from build123d import *

# Parameters (mm, degrees)
SKETCH1_R           = 1.25
BOSS_EXTRUDE1_DEPTH = 10
CHAMFER1_SIZE       = 0.2


with BuildPart() as part:
    # Sketch1 → Boss-Extrude1 (new body)
    with BuildSketch(Plane(origin=(0, 0, 0), x_dir=(1, 0, 0), z_dir=(0, 1, 0))):
        Polygon((1.443375673, 2.5), (-1.443375673, 2.5), (-2.886751346, 0), (-1.443375673, -2.5), (1.443375673, -2.5), (2.886751346, 0), align=None)
        with Locations(Location((0, 0, 0), (0, 0, 270))):  # turned: the seam where the file's is
            Circle(SKETCH1_R, mode=Mode.SUBTRACT)
    extrude(amount=BOSS_EXTRUDE1_DEPTH)

    # Chamfer1
    chamfer1_edges = [part.edges().sort_by_distance(p)[0] for p in [
        (0, 0, -1.25),
        (0, 10, -1.25),
    ]]
    chamfer(chamfer1_edges, length=CHAMFER1_SIZE)

    # Sketch2 → Cut-Revolve1 (revolve, cut)
    with BuildSketch(Plane.XY, mode=Mode.PRIVATE) as cut_revolve1_sk:
        Polygon((2.386751346, 10), (2.886751346, 9.5), (2.886751346, 10), align=None)
        Polygon((2.386751346, 0), (2.886751346, 0), (2.886751346, 0.5), align=None)
    revolve(cut_revolve1_sk.sketch.rotate(Axis((0, 0, 0), (0, 1, 0)), 270), axis=Axis((0, 0, 0), (0, 1, 0)), mode=Mode.SUBTRACT)  # turned: the seam where the file's is


solid = part.part
Read the model definition and answer for the solid it produces. Units are mm, in the model's axes. Coordinates: 2 decimals unless noted, no trailing zeros. Loops run counter-clockwise (first coordinate to the right, second up) from the corner with the lowest first, then second, coordinate; pieces in that order, holes last. Notation, with made-up numbers: (27.25, -1) -> (31.25, -1) arc R18 ccw to (31.25, 24) -> close; hole circle Ø8 at (-37.75, 39.5). An arc over 180 degrees is marked (long way). Answer in a Markdown table with one row per item.
Item 1: For a pull along Z with two mould halves and no side action, classify faces 1 (the flat face through (0, 10, 2)), 2 (the cylindrical face through (-1.22, 4.93, -0.27)), 3 (the flat face through (-2.155, 4.932, -1.268)) as released by +Z, released by -Z, zero draft, split by the parting line, or undercut.
Returned:
| item | result |
|---|---|
| face 1 | zero draft |
| face 2 | undercut |
| face 3 | released by -Z |
Item 2: A cutting plane is placed at B-B on y = 3.5. Determine the outline of the cut face in (x, z), plus the area to 3 significant figures.
Returned:
| item | result |
|---|---|
| outline | (-2.89, 0) -> (-1.44, -2.5) -> (1.44, -2.5) -> (2.89, 0) -> (1.44, 2.5) -> (-1.44, 2.5) -> close; hole circle Ø2.5 at (0, 0) |
| area | 16.7 mm^2 |
Item 3: A cutting plane is placed at A-A on x = 0. Determine the outline of the cut face in (y, z), plus the area to 3 significant figures.
Returned:
| item | result |
|---|---|
| outline | (0, -2.39) -> (0.11, -2.5) -> (9.89, -2.5) -> (10, -2.39) -> (10, -1.45) -> (9.8, -1.25) -> (0.2, -1.25) -> (0, -1.45) -> close; (0, 1.45) -> (0.2, 1.25) -> (9.8, 1.25) -> (10, 1.45) -> (10, 2.39) -> (9.89, 2.5) -> (0.11, 2.5) -> (0, 2.39) -> close |
| area | 24.9 mm^2 |
Item 4: Straight lines are drawn through the part: line 1 along Z through (x, y) = (0.35, 0.75); line 2 along X through (y, z) = (6.5, -0.55); line 3 along X through (y, z) = (9, -1.1). For each, find the intervals that lie inside material, in ascending order. Write a range as [from, to].
Returned:
| item | result |
|---|---|
| line 1 | z = [-2.5, -1.2], [1.2, 2.5] |
| line 2 | x = [-2.57, -1.12], [1.12, 2.57] |
| line 3 | x = [-2.25, -0.59], [0.59, 2.25] |
Item 5: This flat-tipped pin is pushed along its axis until it touches: P1, Ø3, axis at y = 8, z = -0.5, coming from the +X side. Where does it stop, or does it pass through?
Returned:
| item | result |
|---|---|
| P1 | stops at x = 2.89 |
